Design review of the part built by this model. Coordinates are the model's own, in mm. Give positions to 0.01 mm unless a question says otherwise; leave off trailing zeros. Order: outer loops, then holes, each group sorted by start corner. A loop starts at its lowest first (then second) coordinate and runs counter-clockwise, first axis right, second up. Notation, with made-up numbers: (11.5, 9.25) -> (60.5, 9.25) arc R33 cw to (60.5, 47.25) -> close; hole circle Ø1 at (86.5, 68.25). An arc over 180 degrees is marked (long way). One line per item, written item: value.
from build123d import *

# Parameters (mm, degrees)
F0_R     = 1.905
F0_R_2   = 14.2875
F0_R_3   = 4.7625
F1_DEPTH = 12.7
F2_R     = 19.05
F3_DEPTH = 25.4
F4_W     = 431.8
F4_H     = 139.7
F5_DEPTH = 12.7


with BuildPart() as f1:
    # F0 (on Right) → F1 (new body)
    with BuildSketch(Plane.YZ):
        with BuildLine():
            Line((0, 355.6), (0, 0))
            Line((0, 0), (12.7, 0))
            ThreePointArc((12.7, 0), (50.8, 12.7), (88.9, 0))
            Line((88.9, 0), (431.8, 0))
            Line((431.8, 0), (431.8, 355.6))
            Line((431.8, 355.6), (0, 355.6))
        make_face()
        with Locations((61.096733, 42.182442)):
            Circle(F0_R, mode=Mode.SUBTRACT)
        with Locations((228.6, 63.5)):
            Circle(F0_R_2, mode=Mode.SUBTRACT)
        with Locations((330.2, 7.62)):
            Circle(F0_R_3, mode=Mode.SUBTRACT)
        with Locations((330.2, 76.2)):
            Circle(F0_R_2, mode=Mode.SUBTRACT)
        with Locations((114.3, 127)):
            Circle(F0_R_2, mode=Mode.SUBTRACT)
        with Locations((383.379782, 192.465496)):
            Circle(F0_R, mode=Mode.SUBTRACT)
    extrude(amount=F1_DEPTH)

    # F2 (on face) → F3 (cut)
    with BuildSketch(Plane.YZ.offset(12.7)):
        with Locations((152.4, 23.05)):
            Circle(F2_R)
        with Locations((241.3, 23.05)):
            Circle(F2_R)
    extrude(amount=-F3_DEPTH, mode=Mode.SUBTRACT)

    # F4 (on face) → F5 (cut, through all)
    with BuildSketch(Plane.YZ.offset(12.7)):
        with Locations((215.9, 285.75)):
            Rectangle(F4_W, F4_H)
    extrude(amount=-F5_DEPTH, mode=Mode.SUBTRACT)


solid = f1.part
Item 1: To check wall thickness, follow line 1 along Z through (x, y) = (8.75, 330.2); line 2 along Z through (x, y) = (8.5, 228.6); line 3 along Y through (x, z) = (9, 79). State the ranges of each line that lie inside material, in increasing order. Write a range as from..to.
Returned:
line 1: 0..2.86, 12.38..61.91, 90.49..215.9
line 2: 0..8.85, 37.25..49.21, 77.79..215.9
line 3: 0..316.19, 344.21..431.8
Item 2: Draft analysis for pull direction Y (two halves, no side actions). For faces 1 (the flat face through (12.7, 213, 109)), 2 (the cylindrical face through (6.44, 259.47, 28.77)), 3 (the flat face through (6, 0, 109)), state which applies: pulls with the +Y half, pulls with the -Y half, needs draft (parallel to the pull), parting line crosses it, or undercut.
Returned:
face 1: needs draft
face 2: undercut
face 3: pulls with the -Y half
Item 3: Add section B-B on x = 7.5. Count the separate pieces of the cut face and the enclosed holes in it, plus the area to 3 significant figures.
Returned:
separate pieces: 1
enclosed holes: 8
area: 88,300 mm²
Item 4: Add section A-A on y = 228.6. Give the boundary of the cut face in (x, z).
Returned:
outline: (0, 0) -> (12.7, 0) -> (12.7, 8.85) -> (0, 8.85) -> close; (0, 37.25) -> (12.7, 37.25) -> (12.7, 49.21) -> (0, 49.21) -> close; (0, 77.79) -> (12.7, 77.79) -> (12.7, 215.9) -> (0, 215.9) -> close
Item 5: Add section C-C on y = 53. Give the boundary of the cut face in (x, z), plus the area to 3 significant figures.
Returned:
outline: (0, 12.66) -> (12.7, 12.66) -> (12.7, 215.9) -> (0, 215.9) -> close
area: 2,580 mm²
